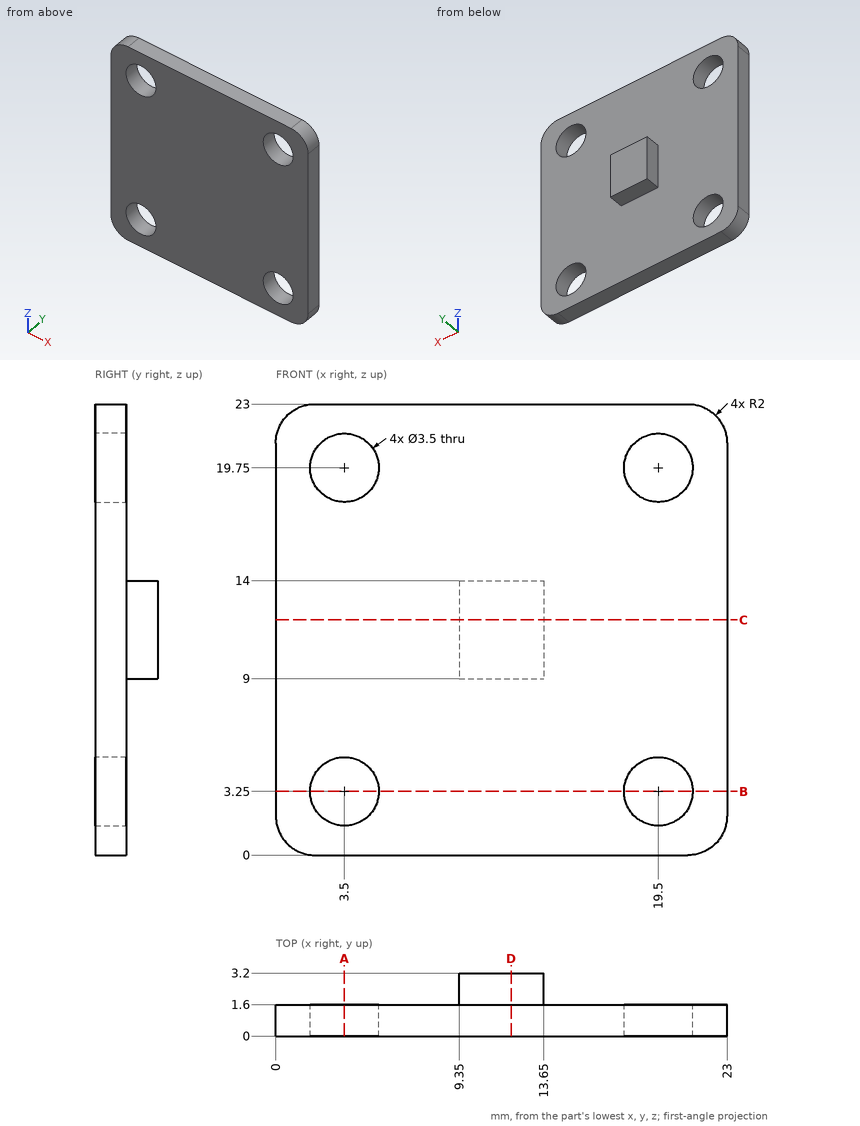
Drawing for the job (mm, zero at the part's lowest x, y, z). Give positions to 0.01 mm unless a question says otherwise; leave off trailing zeros. Loops run counter-clockwise (first coordinate to the right, second up) from the corner with the lowest first, then second, coordinate; pieces in that order, holes last.
1) Band-saw the part on B-B on z = 3.25. List the corners of the cut face in (x, y), then the cut area to 3 significant figures.
Values follow:
outline: (0, 0) - (1.75, 0) - (1.75, 1.6) - (0, 1.6) - close; (5.25, 0) - (17.75, 0) - (17.75, 1.6) - (5.25, 1.6) - close; (21.25, 0) - (23, 0) - (23, 1.6) - (21.25, 1.6) - close
area: 25.6 mm2
2) Probe line 1 along X through (y, z) = (1.2, 19.75); line 2 along X through (y, z) = (0.7, 18.5); line 3 along Z through (x, y) = (3, 0.9). List the from-to ranges inside material, lowest first.
Values follow:
line 1: x = 0 to 1.75, 5.25 to 17.75, 21.25 to 23
line 2: x = 0 to 2.28, 4.72 to 18.28, 20.72 to 23
line 3: z = 0 to 1.57, 4.93 to 18.07, 21.43 to 23
3) Band-saw the part on C-C on z = 12. List the corners of the cut face in (x, y), then the cut area to 3 significant figures.
Values follow:
outline: (0, 0) - (23, 0) - (23, 1.6) - (13.65, 1.6) - (13.65, 3.2) - (9.35, 3.2) - (9.35, 1.6) - (0, 1.6) - close
area: 43.7 mm2
4) Drop flat-ended pins along their axis: P1, Ø0.8, axis at y = 2.5, z = 11.5, coming from the -X side; P2, Ø4.5, axis at x = 19.5, z = 3.25, coming from the +Y side. Give the stop position or say it passes through.
Values follow:
P1: stops at x = 9.35
P2: stops at y = 1.6
5) Band-saw the part on D-D on x = 12. List the corners of the cut face in (y, z).
Values follow:
outline: (0, 0) - (1.6, 0) - (1.6, 9) - (3.2, 9) - (3.2, 14) - (1.6, 14) - (1.6, 23) - (0, 23) - close
6) Band-saw the part on A-A on x = 3.5. List the corners of the cut face in (y, z).
Values follow:
outline: (0, 0) - (1.6, 0) - (1.6, 1.5) - (0, 1.5) - close; (0, 5) - (1.6, 5) - (1.6, 18) - (0, 18) - close; (0, 21.5) - (1.6, 21.5) - (1.6, 23) - (0, 23) - close
